Design review of the part built by this model. Coordinates are the model's own, in mm. Face numbers are marked on the shaded views. A direction names the side the tool comes from. Give positions to 0.01 mm unless a question says otherwise; leave off trailing zeros. Order: outer loops, then holes, each group sorted by start corner. A loop starts at its lowest first (then second) coordinate and runs counter-clockwise, first axis right, second up. Notation, with made-up numbers: (-36.75, 2.25) -> (-11.75, 2.25) arc R36 cw to (-11.75, 37.25) -> close; hole circle Ø4 at (7.5, -0.5). An arc over 180 degrees is marked (long way). One line per item, written item: value.
Autodesk Inventor part; units mm, degrees
ref_plane "YZ Plane" through (0, 0, 0) normal (1, 0, 0) x (0, 1, 0)
ref_plane "XZ Plane" through (0, 0, 0) normal (0, 1, 0) x (-1, 0, 0)
ref_plane "XY Plane" through (0, 0, 0) normal (0, 0, 1) x (1, 0, 0)
sketch "Sketch1" plane through (0, 0, 0) normal (0, 0, 1) x (1, 0, 0)
  line L0 (0, 0) -> (0, 16) construction
  line L1 (-9.5, 0) -> (-9.5, 16)
  line L2 (9.5, 16) -> (9.5, 0)
  arc A0 (-9.5, 0) -> (9.5, 0) centre (0, 0) ccw
  arc A1 (9.5, 16) -> (-9.5, 16) centre (0, 16) ccw
  line L3 (-10.5, 16) -> (-10.5, 0)
  arc A2 (-10.5, 0) -> (10.5, 0) centre (0, 0) ccw
  line L4 (10.5, 0) -> (10.5, 16)
  arc A3 (10.5, 16) -> (-10.5, 16) centre (0, 16) ccw
  point P0 (0, 8)
  dimension "d3" = 9.5
  dimension "d4" = 16
  dimension "d5" = 1
extrude "Extrusion1" add sketch "Sketch1" along normal mid plane 10
properties part number "Colierî"
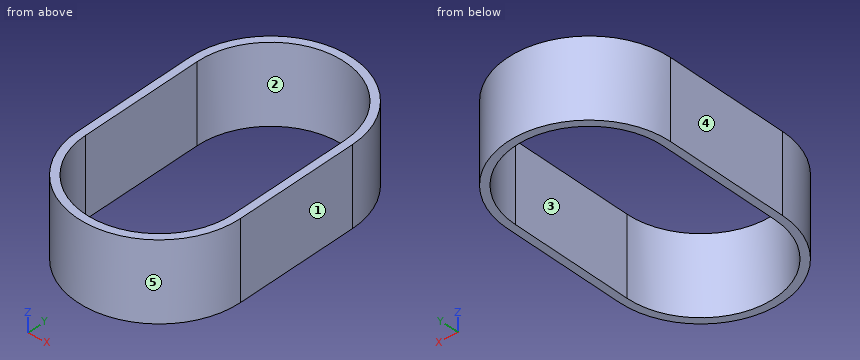
Item 1: Add section C-C on y = 14. Give the boundary of the cut face in (x, z).
Returned:
outline: (-10.5, -5) -> (-9.5, -5) -> (-9.5, 5) -> (-10.5, 5) -> close; (9.5, -5) -> (10.5, -5) -> (10.5, 5) -> (9.5, 5) -> close
Item 2: Add section A-A on x = 0. Give the boundary of the cut face in (y, z), plus the area to 3 significant figures.
Returned:
outline: (-10.5, -5) -> (-9.5, -5) -> (-9.5, 5) -> (-10.5, 5) -> close; (25.5, -5) -> (26.5, -5) -> (26.5, 5) -> (25.5, 5) -> close
area: 20.0 mm²
Item 3: Clearance check with flat-ended pins moving along their axes: P1, Ø4, axis at x = 4, z = 2, coming from the +Y side; P2, Ø1, axis at x = -1, z = 3, coming from the +Y side. State where each tip first meets the part, or that it passes through.
Returned:
P1: y = 26.31
P2: y = 26.49
Item 4: Add section B-B on z = -0.5. Give the boundary of the cut face in (x, y).
Returned:
outline: (-10.5, 0) arc R10.5 ccw to (10.5, 0) -> (10.5, 16) arc R10.5 ccw to (-10.5, 16) -> close; hole (-9.5, 0) arc R9.5 ccw to (9.5, 0) -> (9.5, 16) arc R9.5 ccw to (-9.5, 16) -> close
Item 5: Draft analysis for pull direction Y (two halves, no side actions). For the marked faces 3, 4 and 5, state which applies: pulls with the +Y half, pulls with the -Y half, needs draft (parallel to the pull), parting line crosses it, or undercut.
Returned:
face 3: undercut
face 4: needs draft
face 5: pulls with the -Y half
Item 6: Machinability: for the marked faces 1 and 2, which of the approach directions +Z, -Z, +X, -X, +Y, -Y give a long, thin tool a straight path to every point of the face, cutting with its end or side? Answer none if there is none.
Returned:
face 1: +Z, -Z, +X, +Y, -Y
face 2: +Z, -Z
Item 7: To check wall thickness, follow line 1 along X through (y, z) = (1.5, 3.5); line 2 along Y through (x, z) = (3.5, 4.25); line 3 along X through (y, z) = (-6, 1.25). State the ranges of each line that lie inside material, in increasing order. Write a range as from..to.
Returned:
line 1: -10.5..-9.5, 9.5..10.5
line 2: -9.9..-8.83, 24.83..25.9
line 3: -8.62..-7.37, 7.37..8.62
